```python
from build123d import *

# Parameters (mm, degrees)
CUT_EXTRUDE1_DEPTH = 1
FILLET1_R          = 0.2


with BuildPart() as part:
    # Sketch1 → Revolve1 (revolve)
    with BuildSketch(Plane.XY, mode=Mode.PRIVATE) as revolve1_sk:
        Polygon((0, 0), (0, 14.4), (2.8, 14.4), (2.8, 12), (1.5, 12), (1.5, 0), align=None)
    revolve(revolve1_sk.sketch.rotate(Axis((0, 0, 0), (0, 1, 0)), 90), axis=Axis((0, 0, 0), (0, 1, 0)))

    # Sketch2 → Cut-Extrude1 (cut)
    with BuildSketch(Plane(origin=(0, 14.4, 0), x_dir=(1, 0, 0), z_dir=(0, 1, 0))):
        Polygon((0, -1.443375673), (1.25, -0.721687836), (1.25, 0.721687836), (0, 1.443375673), (-1.25, 0.721687836), (-1.25, -0.721687836), align=None)
    extrude(amount=-CUT_EXTRUDE1_DEPTH, mode=Mode.SUBTRACT)

    # Fillet1
    fillet1_edges = [part.edges().sort_by_distance(p)[0] for p in [
        (0, 14.4, 2.8),
    ]]
    fillet(fillet1_edges, radius=FILLET1_R)


solid = part.part
```
Source: CAD feature listing. Evaluate the final solid. Frame: model axes, mm. A direction names the side the tool comes from. Round coordinates to 2 decimals unless told otherwise and drop trailing zeros. Order: outer loops, then holes, each group sorted by start corner. A loop starts at its lowest first (then second) coordinate and runs counter-clockwise, first axis right, second up. Notation, with made-up numbers: (-0.5, -29.75) -> (32.5, -29.75) arc R32 ccw to (32.5, 6.25) -> close; hole circle Ø5 at (3, -19.5). An arc over 180 degrees is marked (long way). One line per item, written item: value. Start each with the question number.
Q1. Material intervals for probe 1 along Y at (x, z) = (0.75, -0.9); probe 2 along X at (y, z) = (12.25, 2.4); probe 3 along Y at (x, z) = (-2.2, -1.3), sorted ascending.
Q2. Access query for faces 1 (the flat face through (0.616, 13.907, 1.088)), 2 (the flat face through (0, 0, 0)), 3 (the flat face through (1.2, 12, -1.2)). Directions: +Z, -Z, +X, -X, +Y, -Y. A direction counts if a zero-diameter tool reaches every point of the face in a straight line with its end or side. Return the directions, or none.
Q3. Section query B-B (y = 8). Return the cut outline in (x, z).
Q4. Pin query (flat end, axial travel): pin 1 (0.8 mm diameter, centred on y = 14, z = 0.5, fed in from -X); pin 2 (3 mm diameter, centred on x = -2, y = 11.5, fed in from -Z); pin 3 (1 mm diameter, centred on x = -1.5, y = 8.5, fed in from -Z). Return the tip coordinate at first contact, or that it passes through.
Q5. Section query A-A (z = 0). Return the cut outline in (x, y).
Q6. Draft query along X for faces 4 (the cylindrical face through (-0.45, 5.92, -1.43)), 5 (the flat face through (1.1, 14.4, 1.1)), 6 (the flat face through (1.25, 14, 0)), 7 (the flat face through (-0.616, 13.907, -1.088)). Return one class per face: pulls with the +X half, pulls with the -X half, needs draft (parallel to the pull), parting line crosses it, or undercut.
Findings below:
1. probe 1: 0 to 13.4
1. probe 2: -1.44 to 1.44
1. probe 3: 12 to 14.4
2. face 1: +Y
2. face 2: +Z, -Z, +X, -X, -Y
2. face 3: -Y
3. outline: circle Ø3 at (0, 0)
4. pin 1: x = -2.8
4. pin 2: z = -2.74
4. pin 3: z = -1.12
5. outline: (-2.8, 12) -> (-1.5, 12) -> (-1.5, 0) -> (1.5, 0) -> (1.5, 12) -> (2.8, 12) -> (2.8, 14.2) arc R0.2 ccw to (2.6, 14.4) -> (1.25, 14.4) -> (1.25, 13.4) -> (-1.25, 13.4) -> (-1.25, 14.4) -> (-2.6, 14.4) arc R0.2 ccw to (-2.8, 14.2) -> close
6. face 4: parting line crosses it
6. face 5: needs draft
6. face 6: undercut
6. face 7: undercut
